from build123d import *

# Parameters (mm, degrees)
SKETCH3_W           = 234.95
SKETCH3_H           = 30.48
SKETCH3_R           = 1.574999898
SKETCH3_W_2         = 25.4
SKETCH3_H_2         = 3.175
BOSS_EXTRUDE1_DEPTH = 3.175
SKETCH4_W           = 107.95
SKETCH4_H           = 3.175
SKETCH4_W_2         = 12.7
BOSS_EXTRUDE2_DEPTH = 3.175
SKETCH5_W           = 3.175
SKETCH5_H           = 17.78
SKETCH5_W_2         = 3.81
CUT_EXTRUDE1_DEPTH  = 7.62
SKETCH6_R           = 5.969
CUT_EXTRUDE2_DEPTH  = 5.08


with BuildPart() as part:
    # Sketch3 → Boss-Extrude1 (new body)
    # profile 1 of 7: a face of its own
    with BuildSketch(Plane.XY):
        with Locations((-63.5, 8.8475)):
            Rectangle(SKETCH3_W, SKETCH3_H)
        with BuildLine():
            ThreePointArc((-163.6, 17.5), (-162.135533906, 21.035533906), (-158.6, 22.5))
            Line((-158.6, 22.5), (-127, 22.5))
            Line((-127, 22.5), (-101.6, 22.5))
            Line((-101.6, 22.5), (-101.6, 19.325))
            Line((-101.6, 19.325), (-101.6, 3.175))
            Line((-101.6, 3.175), (-101.6, 0))
            Line((-101.6, 0), (-127, 0))
            Line((-127, 0), (-158.6, 0))
            ThreePointArc((-158.6, 0), (-162.135533906, 1.464466094), (-163.6, 5))
            Line((-163.6, 5), (-163.6, 17.5))
        make_face(mode=Mode.SUBTRACT)
        with BuildLine():
            Line((-25.4, 22.5), (0, 22.5))
            Line((0, 22.5), (31.6, 22.5))
            ThreePointArc((31.6, 22.5), (35.135533906, 21.035533906), (36.6, 17.5))
            Line((36.6, 17.5), (36.6, 5))
            ThreePointArc((36.6, 5), (35.135533906, 1.464466094), (31.6, 0))
            Line((31.6, 0), (0, 0))
            Line((0, 0), (-25.4, 0))
            Line((-25.4, 0), (-25.4, 3.175))
            Line((-25.4, 3.175), (-25.4, 19.325))
            Line((-25.4, 19.325), (-25.4, 22.5))
        make_face(mode=Mode.SUBTRACT)
    # profile 2 of 7: a face of its own
    with BuildSketch(Plane.XY):
        with BuildLine():
            ThreePointArc((-158.6, 0), (-162.135533906, 1.464466094), (-163.6, 5))
            Line((-163.6, 5), (-163.6, 17.5))
            ThreePointArc((-163.6, 17.5), (-162.135533906, 21.035533906), (-158.6, 22.5))
            Line((-158.6, 22.5), (-127, 22.5))
            Line((-127, 22.5), (-127, 0))
            Line((-127, 0), (-158.6, 0))
        make_face()
        with Locations((-132.45, 20.25)):
            Circle(SKETCH3_R, mode=Mode.SUBTRACT)
        with Locations((-132.45, 2.250000072)):
            Circle(SKETCH3_R, mode=Mode.SUBTRACT)
        with BuildLine():
            ThreePointArc((-143.175, 11.25), (-141.3, 13.125), (-139.425, 11.25))
            ThreePointArc((-139.425, 11.25), (-141.3, 9.375), (-143.175, 11.25))
        make_face(mode=Mode.SUBTRACT)
        with BuildLine():
            ThreePointArc((-155.35, 11.25), (-152.6, 14), (-149.85, 11.25))
            ThreePointArc((-149.85, 11.25), (-152.6, 8.5), (-155.35, 11.25))
        make_face(mode=Mode.SUBTRACT)
    # profile 3 of 7: a face of its own
    with BuildSketch(Plane.XY):
        with BuildLine():
            Line((36.6, 5), (36.6, 17.5))
            ThreePointArc((36.6, 17.5), (35.135533906, 21.035533906), (31.6, 22.5))
            Line((31.6, 22.5), (0, 22.5))
            Line((0, 22.5), (0, 0))
            Line((0, 0), (31.6, 0))
            ThreePointArc((31.6, 0), (35.135533906, 1.464466094), (36.6, 5))
        make_face()
        with Locations((5.45, 2.250000072)):
            Circle(SKETCH3_R, mode=Mode.SUBTRACT)
        with Locations((5.45, 20.25)):
            Circle(SKETCH3_R, mode=Mode.SUBTRACT)
        with BuildLine():
            ThreePointArc((16.175, 11.25), (14.3, 13.125), (12.425, 11.25))
            ThreePointArc((12.425, 11.25), (14.3, 9.375), (16.175, 11.25))
        make_face(mode=Mode.SUBTRACT)
        with BuildLine():
            ThreePointArc((28.35, 11.25), (25.6, 14), (22.85, 11.25))
            ThreePointArc((22.85, 11.25), (25.6, 8.5), (28.35, 11.25))
        make_face(mode=Mode.SUBTRACT)
    # profile 4 of 7: a face of its own
    with BuildSketch(Plane.XY):
        with Locations((-12.7, 1.5875)):
            Rectangle(SKETCH3_W_2, SKETCH3_H_2)
    # profile 5 of 7: a face of its own
    with BuildSketch(Plane.XY):
        with Locations((-12.7, 20.9125)):
            Rectangle(SKETCH3_W_2, SKETCH3_H_2)
    # profile 6 of 7: a face of its own
    with BuildSketch(Plane.XY):
        with Locations((-114.3, 20.9125)):
            Rectangle(SKETCH3_W_2, SKETCH3_H_2)
    # profile 7 of 7: a face of its own
    with BuildSketch(Plane.XY):
        with Locations((-114.3, 1.5875)):
            Rectangle(SKETCH3_W_2, SKETCH3_H_2)
    extrude(amount=BOSS_EXTRUDE1_DEPTH)

    # Sketch4 → Boss-Extrude2 (add)
    with BuildSketch(Plane.XY.offset(3.175)):
        with Locations((-63.5, 28.85)):
            Rectangle(SKETCH4_W, SKETCH4_H)
        with Locations((-136.525, 28.85)):
            Rectangle(SKETCH4_W_2, SKETCH4_H)
        with Locations((-161.925, 28.85)):
            Rectangle(SKETCH4_W_2, SKETCH4_H)
        Polygon((-142.875, 27.2625), (-155.575, 27.2625), (-168.275, 27.2625), (-180.975, 27.2625), (-180.975, 24.0875), (53.975, 24.0875), (53.975, 27.2625), (41.275, 27.2625), (28.575, 27.2625), (15.875, 27.2625), (3.175, 27.2625), (-9.525, 27.2625), (-117.475, 27.2625), (-130.175, 27.2625), align=None)
        with Locations((9.525, 28.85)):
            Rectangle(SKETCH4_W_2, SKETCH4_H)
        with Locations((34.925, 28.85)):
            Rectangle(SKETCH4_W_2, SKETCH4_H)
        Polygon((53.975, -6.3925), (-180.975, -6.3925), (-180.975, -9.5675), (-168.275, -9.5675), (-155.575, -9.5675), (-142.875, -9.5675), (-130.175, -9.5675), (-117.475, -9.5675), (-9.525, -9.5675), (3.175, -9.5675), (15.875, -9.5675), (28.575, -9.5675), (41.275, -9.5675), (53.975, -9.5675), align=None)
        with Locations((34.925, -11.155)):
            Rectangle(SKETCH4_W_2, SKETCH4_H)
        with Locations((9.525, -11.155)):
            Rectangle(SKETCH4_W_2, SKETCH4_H)
        with Locations((-63.5, -11.155)):
            Rectangle(SKETCH4_W, SKETCH4_H)
        with Locations((-136.525, -11.155)):
            Rectangle(SKETCH4_W_2, SKETCH4_H)
        with Locations((-161.925, -11.155)):
            Rectangle(SKETCH4_W_2, SKETCH4_H)
    extrude(amount=-BOSS_EXTRUDE2_DEPTH)

    # Sketch5 → Cut-Extrude1 (cut)
    with BuildSketch(Plane.XY.offset(3.175)):
        with Locations((-179.3875, 8.8475)):
            Rectangle(SKETCH5_W, SKETCH5_H)
        with Locations((52.07, 8.8475)):
            Rectangle(SKETCH5_W_2, SKETCH5_H)
    extrude(amount=-CUT_EXTRUDE1_DEPTH, mode=Mode.SUBTRACT)

    # Sketch6 → Cut-Extrude2 (cut)
    with BuildSketch(Plane(origin=(0, 0, 0), x_dir=(-1, 0, 0), z_dir=(0, 0, -1))):
        with Locations((82.931, 8.8475)):
            Circle(SKETCH6_R)
    extrude(amount=-CUT_EXTRUDE2_DEPTH, mode=Mode.SUBTRACT)


solid = part.part
Build history of the part. All positions in model axes, mm. Round coordinates to 2 decimals unless told otherwise and drop trailing zeros. Order: outer loops, then holes, each group sorted by start corner. A loop starts at its lowest first (then second) coordinate and runs counter-clockwise, first axis right, second up. Notation, with made-up numbers: M 73,0 L 105,0 A20 ccw 105,17 Z; hole C -38.75,84.5 d11. An arc over 180 degrees is marked long. Use CSV: the item, a comma, the result in double quotes. Start each with the question number.
(1) Cut at A-A on x = -152.6. List the corners of the cut face in (y, z) (1 decimal).
(2) Cut at B-B on x = -106. List the corners of the cut face in (y, z) (1 decimal).
(3) Flat gauge pins, fed straight in: P1, Ø3.5, axis at x = 14.3, y = 11.25, coming from the -Z side; P2, Ø1, axis at y = 15, z = 1.5, coming from the -X side; P3, Ø1.6, axis at x = 46, z = 2, coming from the +Y side; P4, Ø1.6, axis at y = -10.5, z = 2.5, coming from the -X side (3 decimals). Where does each tip first touch, or does it go through?
(4) Mould opens along X. For faces 1 (the face through (28.347, 11.129, 1.565)), 2 (the face through (-65, 9, 0)) say: +X half, -X half, draft (parallel to the pull), parting line (faces both ways), or undercut.
(5) Cut at C-C on z = 1.55. State how many separate pieces and enclosed holes the cut face has, then the cut area to 3 significant figures.
(6) Drill centre lines: probe 1 along X at (y, z) = (-10, 1.2) (3 decimals); probe 2 along Y at (x, z) = (-132.45, 1.75) (1 decimal); probe 3 along X at (y, z) = (16, 0.55) (3 decimals). Where is each one in solid material? Low to high.
Findings:
1,outline,"M -9.6,0 L 8.5,0 L 8.5,3.2 L -9.6,3.2 Z; M 14,0 L 27.3,0 L 27.3,3.2 L 14,3.2 Z"
2,outline,"M -12.7,0 L 3.2,0 L 3.2,3.2 L -12.7,3.2 Z; M 19.3,0 L 30.4,0 L 30.4,3.2 L 19.3,3.2 Z"
3,P1,"passes through"
3,P2,"stops at x = -177.8"
3,P3,"stops at y = 27.26"
3,P4,"stops at x = -168.275"
4,face 1,"undercut"
4,face 2,"draft"
5,separate pieces,"1"
5,enclosed holes,"11"
5,area,"8,500 mm^2"
6,probe 1,"x = -168.275 to -155.575, -142.875 to -130.175, -117.475 to -9.525, 3.175 to 15.875, 28.575 to 41.275"
6,probe 2,"y = -12.7 to 0.7, 3.8 to 18.7, 21.8 to 30.4"
6,probe 3,"x = -177.8 to -127, -101.6 to -25.4, 0 to 50.165"
